```python
from build123d import *

# Parameters (mm, degrees)
SKETCH001_W  = 6
SKETCH001_H  = 6
PAD001_DEPTH = 0.1
FILLET001_R  = 0.3
PAD008_DEPTH = 0.7
FILLET003_R  = 0.29
PAD009_DEPTH = 0.7
FILLET004_R  = 0.29
PAD010_DEPTH = 0.7
FILLET005_R  = 0.29
SKETCH_W     = 6
SKETCH_H     = 6
PAD_DEPTH    = 3.5
FILLET_R     = 0.3
SKETCH004_R  = 0.5
PAD003_DEPTH = 0.6
SKETCH003_R  = 0.5
PAD004_DEPTH = 0.6
SKETCH005_R  = 0.5
PAD002_DEPTH = 0.6
SKETCH002_R  = 0.5
PAD005_DEPTH = 0.6
SKETCH006_R  = 1.75
PAD006_DEPTH = 6
FILLET006_R  = 0.1
PAD007_DEPTH = 0.7
FILLET002_R  = 0.29


with BuildPart() as fillet001:
    # Sketch001 → Pad001 (new body)
    with BuildSketch(Plane.XY.offset(3.5)):
        with Locations((3.15, -2.25)):
            Rectangle(SKETCH001_W, SKETCH001_H)
    extrude(amount=PAD001_DEPTH)

    # Fillet001
    fillet001_edges = [fillet001.edges().sort_by_distance(p)[0] for p in [
        (6.15, -5.25, 3.55),
        (0.15, -5.25, 3.55),
        (6.15, 0.75, 3.55),
        (0.15, 0.75, 3.55),
    ]]
    fillet(fillet001_edges, radius=FILLET001_R)


with BuildPart() as fillet003:
    # Sketch008 → Pad008 (new body)
    with BuildSketch(Plane.XZ.offset(0.35)):
        Polygon((-0.15, 1.5), (0.15, 1.5), (0.15, -0.5), (-0.15, -1.5), (0.15, -2.5), (0.15, -3.5), (-0.15, -3.5), (-0.15, -2.5), (-0.45, -1.5), (-0.15, -0.5), align=None)
    extrude(amount=-PAD008_DEPTH)

    # Fillet003
    fillet003_edges = [fillet003.edges().sort_by_distance(p)[0] for p in [
        (-0.15, 0, -2.5),
        (-0.15, 0, -0.5),
        (-0.45, 0, -1.5),
        (-0.15, 0, 1.5),
        (0.15, 0, -0.5),
        (-0.15, 0, -1.5),
        (0.15, 0, -2.5),
    ]]
    fillet(fillet003_edges, radius=FILLET003_R)


with BuildPart() as fillet004:
    # Sketch009 → Pad009 (new body)
    with BuildSketch(Plane.XZ.offset(4.85)):
        Polygon((6.45, 1.5), (6.15, 1.5), (6.15, -0.5), (6.45, -1.5), (6.15, -2.5), (6.15, -3.5), (6.45, -3.5), (6.45, -2.5), (6.75, -1.5), (6.45, -0.5), align=None)
    extrude(amount=-PAD009_DEPTH)

    # Fillet004
    fillet004_edges = [fillet004.edges().sort_by_distance(p)[0] for p in [
        (6.45, -4.5, -2.5),
        (6.45, -4.5, -0.5),
        (6.75, -4.5, -1.5),
        (6.45, -4.5, 1.5),
        (6.15, -4.5, -0.5),
        (6.45, -4.5, -1.5),
        (6.15, -4.5, -2.5),
    ]]
    fillet(fillet004_edges, radius=FILLET004_R)


with BuildPart() as fillet005:
    # Sketch010 → Pad010 (new body)
    with BuildSketch(Plane.XZ.offset(0.35)):
        Polygon((6.45, 1.5), (6.15, 1.5), (6.15, -0.5), (6.45, -1.5), (6.15, -2.5), (6.15, -3.5), (6.45, -3.5), (6.45, -2.5), (6.75, -1.5), (6.45, -0.5), align=None)
    extrude(amount=-PAD010_DEPTH)

    # Fillet005
    fillet005_edges = [fillet005.edges().sort_by_distance(p)[0] for p in [
        (6.45, 0, -2.5),
        (6.45, 0, -0.5),
        (6.75, 0, -1.5),
        (6.45, 0, 1.5),
        (6.15, 0, -0.5),
        (6.45, 0, -1.5),
        (6.15, 0, -2.5),
    ]]
    fillet(fillet005_edges, radius=FILLET005_R)


with BuildPart() as fillet_body:
    # Sketch → Pad (new body)
    with BuildSketch(Plane.XY):
        with Locations((3.15, -2.25)):
            Rectangle(SKETCH_W, SKETCH_H)
    extrude(amount=PAD_DEPTH)

    # Fillet
    fillet_edges = [fillet_body.edges().sort_by_distance(p)[0] for p in [
        (6.15, 0.75, 1.75),
        (6.15, -5.25, 1.75),
        (0.15, -5.25, 1.75),
        (0.15, 0.75, 1.75),
    ]]
    fillet(fillet_edges, radius=FILLET_R)


with BuildPart() as pad003:
    # Pad003 base: copy of Fillet body
    add(fillet_body.part)

    # Sketch004 → Pad003 (new body)
    with BuildSketch(Plane.XY.offset(3.5)):
        with Locations((5.15, -0.25)):
            Circle(SKETCH004_R)
    extrude(amount=PAD003_DEPTH)


with BuildPart() as pad004:
    # Pad004 base: copy of Fillet body
    add(fillet_body.part)

    # Sketch003 → Pad004 (new body)
    with BuildSketch(Plane.XY.offset(3.5)):
        with Locations((5.15, -4.25)):
            Circle(SKETCH003_R)
    extrude(amount=PAD004_DEPTH)


with BuildPart() as pad002:
    # Pad002 base: copy of Fillet body
    add(fillet_body.part)

    # Sketch005 → Pad002 (new body)
    with BuildSketch(Plane.XY.offset(3.5)):
        with Locations((1.15, -0.25)):
            Circle(SKETCH005_R)
    extrude(amount=PAD002_DEPTH)


with BuildPart() as pad005:
    # Pad005 base: copy of Fillet body
    add(fillet_body.part)

    # Sketch002 → Pad005 (new body)
    with BuildSketch(Plane.XY.offset(3.5)):
        with Locations((1.15, -4.25)):
            Circle(SKETCH002_R)
    extrude(amount=PAD005_DEPTH)


with BuildPart() as fillet006:
    # Pad006 base: copy of Fillet body
    add(fillet_body.part)

    # Sketch006 → Pad006 (new body)
    with BuildSketch(Plane.XY.offset(3.5)):
        with Locations((3.15, -2.25)):
            Circle(SKETCH006_R)
    extrude(amount=PAD006_DEPTH)

    # Fillet006
    fillet006_edges = [fillet006.edges().sort_by_distance(p)[0] for p in [
        (1.4, -2.25, 9.5),
    ]]
    fillet(fillet006_edges, radius=FILLET006_R)


with BuildPart() as obj1:
    # Sketch007 → Pad007 (new body)
    with BuildSketch(Plane.XZ.offset(4.85)):
        Polygon((-0.15, 1.5), (0.15, 1.5), (0.15, -0.5), (-0.15, -1.5), (0.15, -2.5), (0.15, -3.5), (-0.15, -3.5), (-0.15, -2.5), (-0.45, -1.5), (-0.15, -0.5), align=None)
    extrude(amount=-PAD007_DEPTH)

    # Fillet002
    fillet002_edges = [obj1.edges().sort_by_distance(p)[0] for p in [
        (-0.15, -4.5, -2.5),
        (-0.15, -4.5, -0.5),
        (-0.45, -4.5, -1.5),
        (-0.15, -4.5, 1.5),
        (0.15, -4.5, -0.5),
        (-0.15, -4.5, -1.5),
        (0.15, -4.5, -2.5),
    ]]
    fillet(fillet002_edges, radius=FILLET002_R)

    add(fillet001.part)
    add(fillet003.part)
    add(fillet004.part)
    add(fillet005.part)
    add(pad003.part)
    add(pad004.part)
    add(pad002.part)
    add(pad005.part)
    add(fillet006.part)


solid = obj1.part
```
Verification items for the finished model (mm, model axes). A direction names the side the tool comes from. Coordinates: 2 decimals unless noted, no trailing zeros. Loops run counter-clockwise (first coordinate to the right, second up) from the corner with the lowest first, then second, coordinate; pieces in that order, holes last. Notation, with made-up numbers: (26.25, 50) -> (66.25, 50) arc R26 ccw to (66.25, 85) -> close; hole circle Ø5 at (9.25, -11.75). An arc over 180 degrees is marked (long way). Put each result on its own line as item: value.
1. Section check A-A, the plane x = 3.15. Record the boundary of the cut face in (y, z), then the cut area to 3 significant figures.
Result set:
outline: (-5.25, 0) -> (0.75, 0) -> (0.75, 3.6) -> (-0.5, 3.6) -> (-0.5, 9.4) arc R0.1 ccw to (-0.6, 9.5) -> (-3.9, 9.5) arc R0.1 ccw to (-4, 9.4) -> (-4, 3.6) -> (-5.25, 3.6) -> close
area: 42.2 mm^2
2. Gauge pin test, flat ends, axial feed: P1, Ø1.1, axis at x = 1, y = -0.5, coming from the +Z side; P2, Ø0.8, axis at y = 0, z = -3, coming from the -X side; P3, Ø0.6, axis at y = -4.5, z = -3, coming from the +X side. Record the tip position at first contact, or that the pin passes through.
Result set:
P1: stops at z = 4.1
P2: stops at x = -0.15
P3: stops at x = 6.45
3. Tool access check on faces 5 (the face through (3, -2, 0)), 6 (the face through (5.627, -0.1, 3.846)), 7 (the face through (1, -4, 4.1)), 8 (the face through (5, 0, 4.1)), 9 (the face through (1, 0, 4.1)). Record the directions out of +Z, -Z, +X, -X, +Y, -Y that give a thin tool (end or side, any length) a straight path to the whole face; none if there is none.
Result set:
face 5: -Z, +Y, -Y
face 6: +Z
face 7: +Z, -X, -Y
face 8: +Z, +X, +Y
face 9: +Z, -X, +Y
4. Section check B-B, the plane z = -0.25. Record the boundary of the cut face in (x, y), then the cut area to 3 significant figures.
Result set:
outline: (-0.15, -4.85) -> (0.15, -4.85) -> (0.15, -4.15) -> (-0.15, -4.15) -> close; (-0.15, -0.35) -> (0.15, -0.35) -> (0.15, 0.35) -> (-0.15, 0.35) -> close; (6.15, -4.85) -> (6.45, -4.85) -> (6.45, -4.15) -> (6.15, -4.15) -> close; (6.15, -0.35) -> (6.45, -0.35) -> (6.45, 0.35) -> (6.15, 0.35) -> close
area: 0.840 mm^2
5. Mould release check, pull along X, two halves, no side actions. Record for faces 1 (the face through (0.15, -2, 2)), 2 (the face through (5.627, -4.1, 3.846)), 3 (the face through (1.627, -0.1, 3.846)), 4 (the face through (6.15, -2, 2)): pulls with the +X half, pulls with the -X half, needs draft (parallel to the pull), parting line crosses it, or undercut.
Result set:
face 1: pulls with the -X half
face 2: undercut
face 3: undercut
face 4: pulls with the +X half
6. Section check D-D, the plane y = -2.25. Record the boundary of the cut face in (x, z).
Result set:
outline: (0.15, 0) -> (6.15, 0) -> (6.15, 3.6) -> (4.9, 3.6) -> (4.9, 9.4) arc R0.1 ccw to (4.8, 9.5) -> (1.5, 9.5) arc R0.1 ccw to (1.4, 9.4) -> (1.4, 3.6) -> (0.15, 3.6) -> close
7. Section check C-C, the plane z = 3. Record the boundary of the cut face in (x, y).
Result set:
outline: (0.15, -4.95) arc R0.3 ccw to (0.45, -5.25) -> (5.85, -5.25) arc R0.3 ccw to (6.15, -4.95) -> (6.15, 0.45) arc R0.3 ccw to (5.85, 0.75) -> (0.45, 0.75) arc R0.3 ccw to (0.15, 0.45) -> close
8. Thickness scan on line 1 (Z direction, x = 3.5, y = -0.9); line 2 (X direction, y = -4.9, z = 3); line 3 (Z direction, x = 1, y = -1.1). Record the ranges inside material, lowest first.
Result set:
line 1: z = 0 to 9.5
line 2: x = 0.15 to 6.15
line 3: z = 0 to 3.6
